Design review of the part shown in the three views and the two pictorial views. Dimensions are in mm from the part's minimum x, y and z. Coordinates: 2 decimals unless noted, no trailing zeros. Loops run counter-clockwise (first coordinate to the right, second up) from the corner with the lowest first, then second, coordinate; pieces in that order, holes last. Notation, with made-up numbers: (-22.5, 19) -> (-17.5, 19) arc R25 cw to (-17.5, 41) -> close; hole circle Ø11 at (-34, 66). An arc over 180 degrees is marked (long way). One line per item, written item: value. Start each with the question number.
1. Draft analysis for pull direction X (two halves, no side actions). For the marked faces 1, 2, 3 and 4, state which applies: pulls with the +X half, pulls with the -X half, needs draft (parallel to the pull), parting line crosses it, or undercut.
2. For probe 1 along X at (y, z) = (2.5, 76.5); probe 2 along X at (y, z) = (6.25, 32.5); probe 3 along Z at (x, y) = (32.5, 8.25), list the stretches that pass through material, from the lowest coordinate up.
3. Add section D-D on y = 4. Write out the cut boundary in (x, z).
4. Insertion check: pin 1 (12 mm diameter, centred on x = 32.5, z = 32.5, fed in from -Y); pin 2 (2 mm diameter, centred on y = 6.5, z = 25, fed in from -X); pin 3 (1.5 mm diameter, centred on y = 6, z = 12.5, fed in from +X); pin 4 (2 mm diameter, centred on y = 4.5, z = 13, fed in from -X). Each pin has a flat end and moves straight along its axis. Give the tip position at first contact, or say it passes through.
5. Add section C-C on z = 76.5. Write out the cut boundary in (x, y) (1 decimal).
6. Add section A-A on x = 25.5. Write out the cut boundary in (y, z).
7. Add section B-B on y = 11. Write out the cut boundary in (x, z).
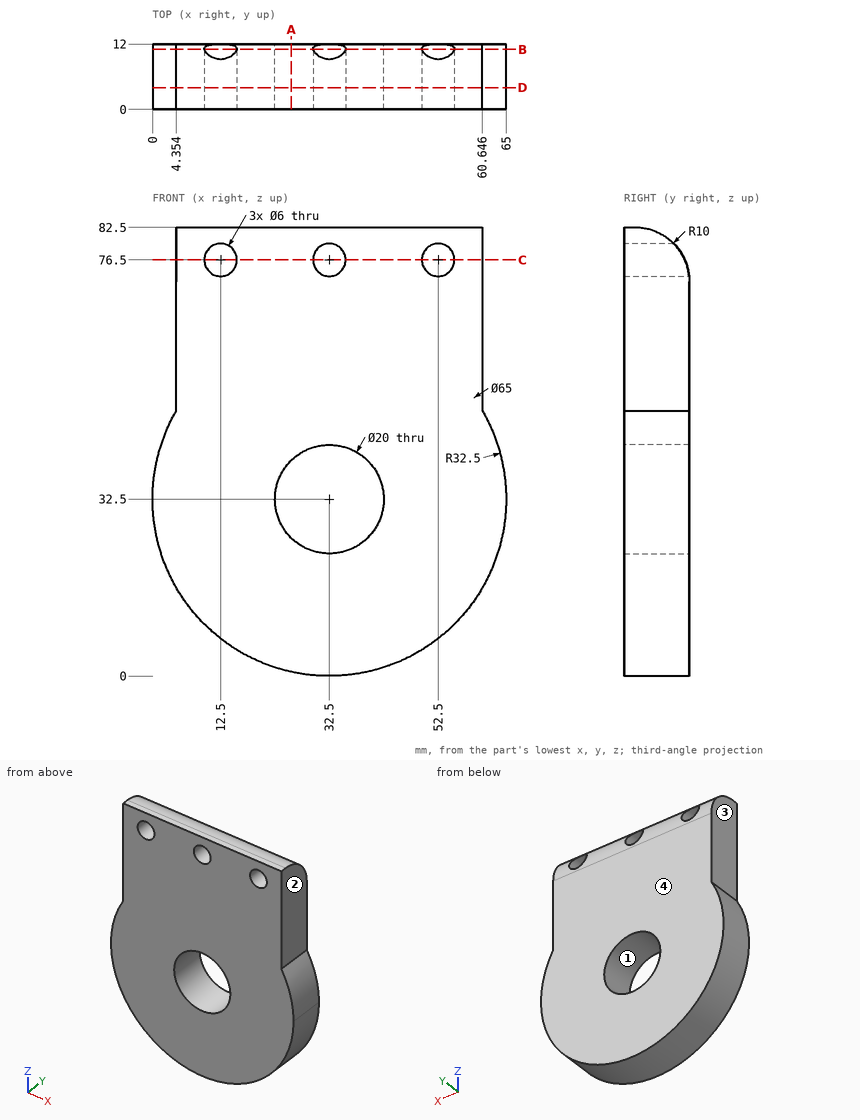
Worked answers:
1. face 1: undercut
1. face 2: pulls with the +X half
1. face 3: pulls with the -X half
1. face 4: needs draft
2. probe 1: x = 4.35 to 9.5, 15.5 to 29.5, 35.5 to 49.5, 55.5 to 60.65
2. probe 2: x = 0 to 22.5, 42.5 to 65
2. probe 3: z = 0 to 22.5, 42.5 to 73.5, 79.5 to 80.31
3. outline: (4.35, 48.75) arc R32.5 ccw (long way) to (60.65, 48.75) -> (60.65, 82.3) -> (4.35, 82.3) -> close; hole circle Ø6 at (12.5, 76.5); hole circle Ø20 at (32.5, 32.5); hole circle Ø6 at (32.5, 76.5); hole circle Ø6 at (52.5, 76.5)
4. pin 1: passes through
4. pin 2: stops at x = 0.66
4. pin 3: stops at x = 58.69
4. pin 4: stops at x = 5.78
5. outline: (4.4, 0) -> (9.5, 0) -> (9.5, 11.2) -> (4.4, 11.2) -> close; (15.5, 0) -> (29.5, 0) -> (29.5, 11.2) -> (15.5, 11.2) -> close; (35.5, 0) -> (49.5, 0) -> (49.5, 11.2) -> (35.5, 11.2) -> close; (55.5, 0) -> (60.6, 0) -> (60.6, 11.2) -> (55.5, 11.2) -> close
6. outline: (0, 0.76) -> (12, 0.76) -> (12, 25.36) -> (0, 25.36) -> close; (0, 39.64) -> (12, 39.64) -> (12, 72.5) arc R10 ccw to (2, 82.5) -> (0, 82.5) -> close
7. outline: (4.35, 48.75) arc R32.5 ccw (long way) to (60.65, 48.75) -> (60.65, 76.86) -> (55.48, 76.86) arc R3 cw (long way) to (49.52, 76.86) -> (35.48, 76.86) arc R3 cw (long way) to (29.52, 76.86) -> (15.48, 76.86) arc R3 cw (long way) to (9.52, 76.86) -> (4.35, 76.86) -> close; hole circle Ø20 at (32.5, 32.5)
